from build123d import *

# Parameters (mm, degrees)
BOSS_EXTRUDE1_DEPTH     = 14
SKETCH4_W               = 28
SKETCH4_H               = 51
BOSS_EXTRUDE2_DEPTH     = 5
SKETCH3_R               = 8
CUT_EXTRUDE1_DEPTH      = 50.099012473
CUT_EXTRUDE3_DEPTH      = 11
CUT_EXTRUDE4_DEPTH      = 49.798206602
CUT_EXTRUDE4_DEPTH_BACK = 49.798206602
SKETCH7_W               = 22
SKETCH7_H               = 15.296617448
BOSS_EXTRUDE3_DEPTH     = 17
CUT_EXTRUDE5_DEPTH      = 63.42802941
CUT_EXTRUDE5_DEPTH_BACK = 63.42802941
SKETCH11_R              = 3


with BuildPart() as part:
    # Sketch1 → Boss-Extrude1 (new, symmetric)
    with BuildSketch(Plane(origin=(0, 0, 0), x_dir=(0, 0, -1), z_dir=(1, 0, 0))):
        Polygon((-13.807105756, -7.671099373), (13.310075259, 43.328900627), (13.310075259, -7.671099373), align=None)
    extrude(amount=BOSS_EXTRUDE1_DEPTH, both=True)

    # Sketch4 → Boss-Extrude2 (add)
    with BuildSketch(Plane(origin=(0, 0, -13.310075259), x_dir=(-1, 0, 0), z_dir=(0, 0, -1))):
        with Locations((0, 17.828900627)):
            Rectangle(SKETCH4_W, SKETCH4_H)
    extrude(amount=BOSS_EXTRUDE2_DEPTH)

    # Sketch3 → Cut-Extrude1 (cut, through all)
    with BuildSketch(Plane(origin=(0, 4.032567199, 7.584155854), x_dir=(1, 0, 0), z_dir=(0, 0.46947156278589475, 0.8829475928589249))):
        with Locations(Location((0, 23.97057959, 0), (0, 0, 270))):
            Circle(SKETCH3_R)
    extrude(amount=-CUT_EXTRUDE1_DEPTH, mode=Mode.SUBTRACT)

    # Sketch6 → Cut-Extrude3 (cut, symmetric)
    with BuildSketch(Plane(origin=(0, 0, 0), x_dir=(0, 0, -1), z_dir=(1, 0, 0))):
        Polygon((18.310075259, 37.822151676), (0.763812466, 4.822430874), (0.763812466, -14.665024569), (18.310075259, -14.665024569), (18.310075259, 4.822430874), align=None)
    extrude(amount=CUT_EXTRUDE3_DEPTH, both=True, mode=Mode.SUBTRACT)

    # Sketch7 → Cut-Extrude4 (cut, two sides: drawn at the far end of the back side and taken through both)
    with BuildSketch(Plane(origin=(0, 0, -0.763812466), x_dir=(-1, 0, 0), z_dir=(0, 0, -1)).offset(-CUT_EXTRUDE4_DEPTH_BACK)):
        with Locations((0, -0.022790649)):
            Rectangle(SKETCH7_W, SKETCH7_H)
    extrude(amount=CUT_EXTRUDE4_DEPTH + CUT_EXTRUDE4_DEPTH_BACK, mode=Mode.SUBTRACT)

    # Sketch10 → Boss-Extrude3 (add)
    with BuildSketch(Plane(origin=(14, 0, 0), x_dir=(0, 0, -1), z_dir=(1, 0, 0))):
        Polygon((-13.807105756, -7.671099373), (-11.680268029, -3.671099373), (18.310075259, -3.671099373), (18.310075259, -7.671099373), align=None)
    boss_extrude3 = extrude(amount=BOSS_EXTRUDE3_DEPTH)

    # Mirror5: Boss-Extrude3 across plane
    add(boss_extrude3.mirror(Plane(origin=(0, 0, 0), x_dir=(0, 0, 1), z_dir=(1, 0, 0))))

    # Sketch11 → Cut-Extrude5 (cut, two sides: drawn at the far end of the back side and taken through both)
    with BuildSketch(Plane.XZ.offset(7.671099373).offset(-CUT_EXTRUDE5_DEPTH_BACK)):
        with Locations(Location((22, 2.807105756, 0), (0, 0, 270))):
            Circle(SKETCH11_R)
        with Locations(Location((-22, 2.807105756, 0), (0, 0, 90))):
            Circle(SKETCH11_R)
    extrude(amount=CUT_EXTRUDE5_DEPTH + CUT_EXTRUDE5_DEPTH_BACK, mode=Mode.SUBTRACT)


solid = part.part
Design review of the part built by this model. Coordinates are the model's own, in mm. A direction names the side the tool comes from. Coordinates: 2 decimals unless noted, no trailing zeros. Order: outer loops, then holes, each group sorted by start corner. A loop starts at its lowest first (then second) coordinate and runs counter-clockwise, first axis right, second up. Notation, with made-up numbers: (81, 60.25) -> (87, 60.25) arc R36 ccw to (87, 96.25) -> close; hole circle Ø4 at (8.5, 74.5). An arc over 180 degrees is marked (long way). Use one line per item in the form item = value. Start each with the question number.
(1) For faces 1 (the flat face through (-14, 14, -6)), 2 (the flat face through (22, -3.671, -3)), 3 (the flat face through (-11, 5, -6)), list the 3-axis set-ups (+Z, -Z, +X, -X, +Y, -Y) from which the entire face can be reached by the end or side of a thin tool; tool diameter is ignored.
(2) Add section A-A on x = -22. State the section outline as (y, z) points.
(3) Add section D-D on x = -9.5. State the section outline as (y, z) points.
(4) Add section B-B on z = 2.5. State the section outline as (x, y) points.
(5) The part is to be moulded in two halves that separate along Z. For faces 4 (the flat face through (-11.3, 17.9, -18.31)), 5 (the cylindrical face through (19.07, -5.64, 3.46)), 6 (the flat face through (0, 7.626, 2)), say which applies: +Z half, -Z half, draft (parallel to the pull), parting line (faces both ways), or undercut.
(6) For probe 1 along X at (y, z) = (3, -6); probe 2 along Y at (x, z) = (19.5, -12.5); probe 3 along Z at (x, y) = (22, -5), list the stretches that pass through material, from the lowest coordinate up.
(7) Insertion check: pin 1 (4 mm diameter, centred on x = -0.5, y = 9, fed in from +Z); pin 2 (15 mm diameter, centred on y = 31.5, z = -3, fed in from +X); pin 3 (15 mm diameter, centred on y = 20, z = -5, fed in from -X). Each pin has a flat end and moves straight along its axis. Give the tip position at first contact, or say it passes through.
(8) Add section C-C on y = 2.5. State the section outline as (x, z) points.
Answer block:
q1.face_1 = +Z, -Z, -X, +Y
q1.face_2 = +Z, -Z, +X, +Y
q1.face_3 = -Z, -Y
q2.outline = (-7.67, -18.31) -> (-3.67, -18.31) -> (-3.67, -0.19) -> (-7.67, -0.19) -> close; (-7.67, 5.81) -> (-3.67, 5.81) -> (-3.67, 11.68) -> (-7.67, 13.81) -> close
q3.outline = (7.63, -2.25) -> (37.82, -18.31) -> (43.33, -18.31) -> (43.33, -13.31) -> (7.63, 5.67) -> close
q4.outline = (-31, -7.67) -> (-24.98, -7.67) -> (-24.98, -3.67) -> (-31, -3.67) -> close; (-19.02, -7.67) -> (-11, -7.67) -> (-11, 7.63) -> (11, 7.63) -> (11, -7.67) -> (19.02, -7.67) -> (19.02, -3.67) -> (14, -3.67) -> (14, 13.59) -> (-14, 13.59) -> (-14, -3.67) -> (-19.02, -3.67) -> close; (24.98, -7.67) -> (31, -7.67) -> (31, -3.67) -> (24.98, -3.67) -> close
q5.face_4 = -Z half
q5.face_5 = undercut
q5.face_6 = draft
q6.probe_1 = -14 to -11, 11 to 14
q6.probe_2 = -7.67 to -3.67
q6.probe_3 = -18.31 to -0.19, 5.81 to 12.39
q7.pin_1 = 5.67
q7.pin_2 = 14
q7.pin_3 = -14
q8.outline = (-14, -18.31) -> (-11, -18.31) -> (-11, 8.4) -> (-14, 8.4) -> close; (11, -18.31) -> (14, -18.31) -> (14, 8.4) -> (11, 8.4) -> close
